Here's how the part is built. I have some questions about the finished solid (model axes, mm). Round coordinates to 2 decimals unless told otherwise and drop trailing zeros. Loops run counter-clockwise (first coordinate to the right, second up) from the corner with the lowest first, then second, coordinate; pieces in that order, holes last. Notation, with made-up numbers: M -5.75,16.5 L 39.25,16.5 A15 cw 39.25,20.5 Z; hole C -7.5,67.5 d11. An arc over 180 degrees is marked long. Answer as a JSON object with one key per item and string values.
Solid Edge part; units mm, degrees
sketch "Sketch1" plane through (0, 0, 0) normal (-1, 0, 0) x (0, -1, 0)
  line L0 (-20, 0) -> (20, 0)
  line L1 (20, 0) -> (20, 390)
  line L2 (20, 390) -> (-20, 390)
  line L3 (-20, 390) -> (-20, 0)
extrude "Protrusion1" add sketch "Sketch1" along normal mid plane 60
sketch "Sketch2" plane through (-30, 0, 187.5) normal (-1, 0, 0) x (0, 0, -1)
  circle A0 centre (-172.5, 0) radius 10.5
extrude "ExtrudedCutout_1" cut sketch "Sketch2" against normal blind 60
sketch "Sketch3" plane through (-30, 0, 187.5) normal (-1, 0, 0) x (0, 0, 1)
  line L0 (202.5, -20) -> (172.5, -20)
  line L1 (202.5, 20) -> (202.5, -20)
  line L2 (172.5, 20) -> (202.5, 20)
  arc A0 (172.5, 20) -> (172.5, -20) centre (172.5, 0) cw
extrude "ExtrudedCutout_2" cut sketch "Sketch3" against normal blind 60
extrude "ExtrudedCutout_3" [suppressed]
sketch "Sketch4" plane through (0, 0, 0) normal (0, 0, -1) x (0, -1, 0)
  line L0 (-20, 30) -> (20, 30)
  line L1 (20, 30) -> (20, -30)
  line L2 (20, -30) -> (-20, -30)
  line L3 (-20, -30) -> (-20, 30)
extrude "ExtrudedCutout_9" cut sketch "Sketch4" against normal blind 10
sketch "Sketch5" plane through (0, -20, 185) normal (0, -1, 0) x (0, 0, 1)
  line L0 (115, -10.5) -> (195, -10.5)
  line L1 (195, -10.5) -> (195, 10.5)
  line L2 (195, 10.5) -> (115, 10.5)
  line L3 (115, 10.5) -> (115, -10.5)
extrude "ExtrudedCutout_11" cut sketch "Sketch5" against normal blind 40
sketch "Sketch6" plane through (-30, 0, 195) normal (-1, 0, 0) x (0, 0, -1)
  circle A0 centre (-165.84, 15.89) radius 2.5
extrude "ExtrudedCutout_13" cut sketch "Sketch6" against normal blind 60
hole "Hole_1" at (15, 0, 10) direction (0, 0, 1) diameter 17.5 depth 95.3 tip angle 118
hole "Hole1" at (-15, 0, 10) direction (0, 0, 1) diameter 17.5 depth 95.3 tip angle 118
hole "Hole_3" at (15, 20, 170) direction (0, -1, 0) diameter 11 end up to next
hole "Hole2" at (-15, 20, 170) direction (0, -1, 0) diameter 11 end up to next
hole "Hole3" at (15, 20, 265) direction (0, -1, 0) diameter 11 end up to next
hole "Hole4" at (-15, 20, 265) direction (0, -1, 0) diameter 11 end up to next
properties material "Steel - Stainless:1.4301 , X5CrNi18-10"
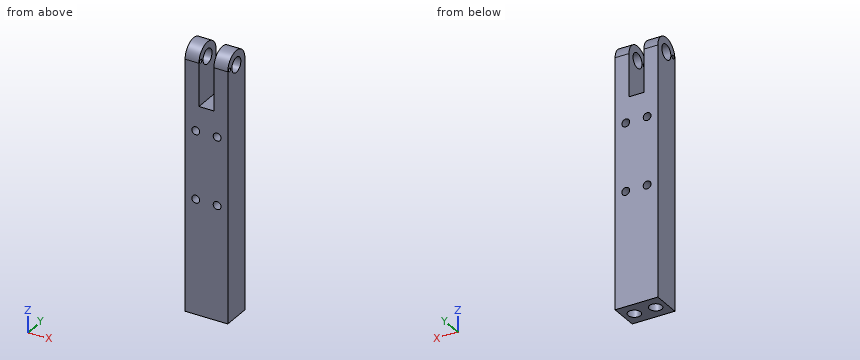
Item 1: I want a section at C-C, the plane y = 5. State how many separate pieces and enclosed holes the cut face has, then the cut area to 3 significant figures.
Resolved:
{"separate pieces": "3", "enclosed holes": "4", "area": "16,600 mm²"}
Item 2: Please list where these lines run through material, in increasing order: probe 1 along Y at (x, z) = (22.25, 360.84); probe 2 along X at (y, z) = (2, 265); probe 3 along Z at (x, y) = (15, -5). Write a range as from..to.
Resolved:
{"probe 1": "-19.98..-18.39, -13.39..-10.47, 10.47..19.98", "probe 2": "-30..-20.5, -9.5..9.5, 20.5..30", "probe 3": "107.55..164.5, 175.5..259.5, 270.5..350.77, 369.23..379.36"}
Item 3: I want a section at B-B, the plane z = 40.5. Please give me the cut outline in (x, y), then the cut area to 3 significant figures.
Resolved:
{"outline": "M -30,-20 L 30,-20 L 30,20 L -30,20 Z; hole C -15,0 d17.5; hole C 15,0 d17.5", "area": "1,920 mm²"}
Item 4: I want a section at A-A, the plane z = 170. Please give me the cut outline in (x, y).
Resolved:
{"outline": "M -30,-20 L -20.5,-20 L -20.5,20 L -30,20 Z; M -9.5,-20 L 9.5,-20 L 9.5,20 L -9.5,20 Z; M 20.5,-20 L 30,-20 L 30,20 L 20.5,20 Z"}
Item 5: I'm going to push flat-ended pins straight in: pin 1 Ø17 at (y, z) = (0, 360) entering from -X; pin 2 Ø3 at (x, y) = (5.5, -8) entering from +Z; pin 3 Ø17 at (x, y) = (-4, -4) entering from +Z; pin 4 Ø4 at (x, y) = (12.5, -12.5) entering from +Z. Where does each tip first touch, or does it pass through?
Resolved:
{"pin 1": "through", "pin 2": "z = 300", "pin 3": "z = 380", "pin 4": "z = 377.02"}
